Source: CAD feature listing. Evaluate the final solid. Frame: model axes, mm. Face numbers are marked on the shaded views. A direction names the side the tool comes from. Round coordinates to 2 decimals unless told otherwise and drop trailing zeros. Loops run counter-clockwise (first coordinate to the right, second up) from the corner with the lowest first, then second, coordinate; pieces in that order, holes last. Notation, with made-up numbers: M 63.5,52.25 L 78.5,52.25 A9 cw 78.5,60.25 Z; hole C 57.5,42.5 d8. An arc over 180 degrees is marked long. One line per item, written item: value.
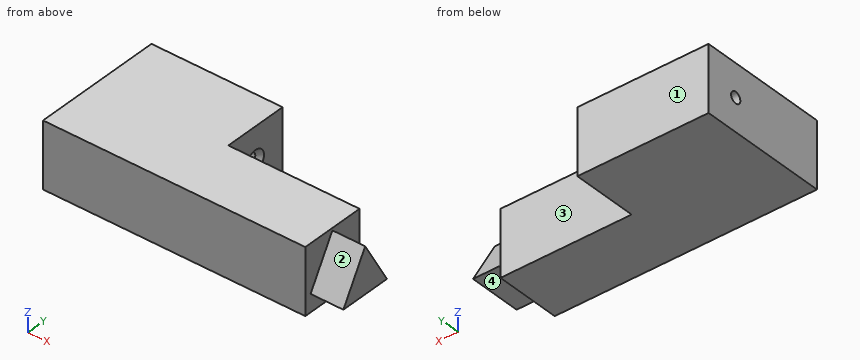
from build123d import *

# Parameters (mm, degrees)
SKETCH_1_W                  = 20
SKETCH_1_H                  = 40
EXTRUDE_1_DEPTH             = 40
SKETCH_16_W                 = 20
SKETCH_16_H                 = 20
EXTRUDE_2_DEPTH             = 40
HOLE_WIZARD_M31_D           = 3.4
HOLE_WIZARD_M31_CSINK_D     = 6.3
HOLE_WIZARD_M31_CSINK_ANGLE = 90
EXTRUDE_3_DEPTH             = 10


with BuildPart() as part:
    # Эскиз1 → Бобышка-Вытянуть1 (new body)
    with BuildSketch(Plane(origin=(0, 0, 0), x_dir=(0, 0, -1), z_dir=(1, 0, 0))):
        with Locations((-27.72412662, 2.360988518)):
            Rectangle(SKETCH_1_W, SKETCH_1_H)
    extrude(amount=EXTRUDE_1_DEPTH)

    # Эскиз16 → Бобышка-Вытянуть2 (add)
    with BuildSketch(Plane(origin=(40, 0, 0), x_dir=(0, 0, -1), z_dir=(1, 0, 0))):
        with Locations((-27.72412662, -7.639011482)):
            Rectangle(SKETCH_16_W, SKETCH_16_H)
    extrude(amount=EXTRUDE_2_DEPTH)

    # Зенковка для винта с полупотайной головкой M31 (through all)
    with Locations(Plane(origin=(40, 0, 0), x_dir=(0, 0, -1), z_dir=(1, 0, 0))):
        with Locations((-27.717933157, 12.344098424)):
            CounterSinkHole(HOLE_WIZARD_M31_D / 2, HOLE_WIZARD_M31_CSINK_D / 2, counter_sink_angle=HOLE_WIZARD_M31_CSINK_ANGLE)

    # Эскиз19 → Бобышка-Вытянуть3 (add)
    with BuildSketch(Plane(origin=(80, 0, 0), x_dir=(0, 0, -1), z_dir=(1, 0, 0))):
        Polygon((-37.01304766, -7.639011482), (-23.0796661, -15.683453077), (-23.0796661, 0.405430112), align=None)
    extrude(amount=EXTRUDE_3_DEPTH)


solid = part.part
1. Reachability of the marked faces 1, 2, 3 and 4 from +Z, -Z, +X, -X, +Y, -Y: full face, straight path, thin tool, end or side. Return the list, or none.
Report:
face 1: +Z, -Z, +X, -X, +Y
face 2: +Z, +X, -Y
face 3: +Z, -Z, +X, +Y
face 4: -Z, +X, +Y, -Y
2. Section query D-D (z = 31.75). Return the cut outline in (x, y).
Report:
outline: M 0,-17.64 L 80,-17.64 L 80,-10.68 L 90,-10.68 L 90,-4.6 L 80,-4.6 L 80,2.36 L 40,2.36 L 40,22.36 L 0,22.36 Z
3. Section query C-C (x = 84.5). Return the cut outline in (y, z), and give its area (3 significant figures).
Report:
outline: M -15.68,23.08 L 0.41,23.08 L -7.64,37.01 Z
area: 112 mm2
4. Pin query (flat end, axial travel): pin 1 (6 mm diameter, centred on y = 16, z = 23, fed in from +X); pin 2 (4.5 mm diameter, centred on y = 12.34, z = 27.72, fed in from +X); pin 3 (3 mm diameter, centred on x = 85, y = -7.5, fed in from -Z). Return the tip coordinate at first contact, or that it passes through.
Report:
pin 1: stops at x = 40
pin 2: stops at x = 39.1
pin 3: stops at z = 23.08
5. Section query B-B (y = -5.5). Return the cut outline in (x, z), and give its area (3 significant figures).
Report:
outline: M 0,17.72 L 80,17.72 L 80,23.08 L 90,23.08 L 90,33.31 L 80,33.31 L 80,37.72 L 0,37.72 Z
area: 1,700 mm2
6. Section query A-A (z = 22.25). Return the cut outline in (x, y), and give its area (3 significant figures).
Report:
outline: M 0,-17.64 L 80,-17.64 L 80,2.36 L 40,2.36 L 40,22.36 L 0,22.36 Z
area: 2,400 mm2
7. Ray query, line 1 (X direction, y = 13, z = 22); line 2 (Y direction, x = 51, z = 26.75); line 3 (X direction, y = -14, z = 27.5). Return the intervals inside material, ascending. Write a range as [from, to].
Report:
line 1: x = [0, 40]
line 2: y = [-17.64, 2.36]
line 3: x = [0, 80]
